For this review, take the finished solid that the model builds, in its own axes (mm). Face numbers are marked on the shaded views. A direction names the side the tool comes from. Coordinates: 2 decimals unless noted, no trailing zeros. Order: outer loops, then holes, each group sorted by start corner. A loop starts at its lowest first (then second) coordinate and runs counter-clockwise, first axis right, second up. Notation, with made-up numbers: M -18.5,33.5 L 12.5,33.5 A16 ccw 12.5,58.5 Z; hole C 30.5,-14 d5. An arc over 180 degrees is marked long. Use CSV: the item, a comma, the result in double quotes.
```python
from build123d import *

# Parameters (mm, degrees)
F0_R     = 15.875
F0_R_2   = 6.35
F1_DEPTH = 31.75
F2_DEPTH = 76.2
F3_R     = 4.445
F4_DEPTH = 76.2


with BuildPart() as f1:
    # F0 (on Top) → F1 (new body)
    with BuildSketch(Plane.XY):
        Circle(F0_R)
        Circle(F0_R_2, mode=Mode.SUBTRACT)
    extrude(amount=-F1_DEPTH)

    # F0 (on Top) → F2 (join)
    with BuildSketch(Plane.XY):
        Circle(F0_R_2)
    extrude(amount=-F2_DEPTH)

    # F3 (on Right) → F4 (join, symmetric)
    with BuildSketch(Plane.YZ):
        with Locations((0, -15.875)):
            Circle(F3_R)
    extrude(amount=F4_DEPTH, both=True)

    # F7 (on Front) → F8 (revolve)
    with BuildSketch(Plane.XZ):
        with BuildLine():
            Line((73.423605, -5.542184), (73.423605, -25.862184))
            ThreePointArc((73.423605, -25.862184), (83.583605, -15.702184), (73.423605, -5.542184))
        make_face()
    revolve(axis=Axis((73.423605, 0, -26.137914), (0, 0, -1)))



with BuildPart() as f6:
    # F5 (on Front) → F6 (revolve)
    with BuildSketch(Plane.XZ):
        with BuildLine():
            Line((-76.2, -26.452393), (-76.2, -6.132393))
            ThreePointArc((-76.2, -6.132393), (-86.36, -16.292393), (-76.2, -26.452393))
        make_face()
    revolve(axis=Axis((-76.2, 0, -32.181646), (0, 0, -1)))


with BuildPart() as f1_1:
    add(f1.part)

    add(f6.part)  # F9 merges F6
    # F5 (on Front) → F9 (revolve)
    with BuildSketch(Plane.XZ):
        with BuildLine():
            Line((-76.2, -26.452393), (-76.2, -6.132393))
            ThreePointArc((-76.2, -6.132393), (-86.36, -16.292393), (-76.2, -26.452393))
        make_face()
    revolve(axis=Axis((-76.2, 0, -32.181646), (0, 0, -1)))


solid = f1_1.part
```
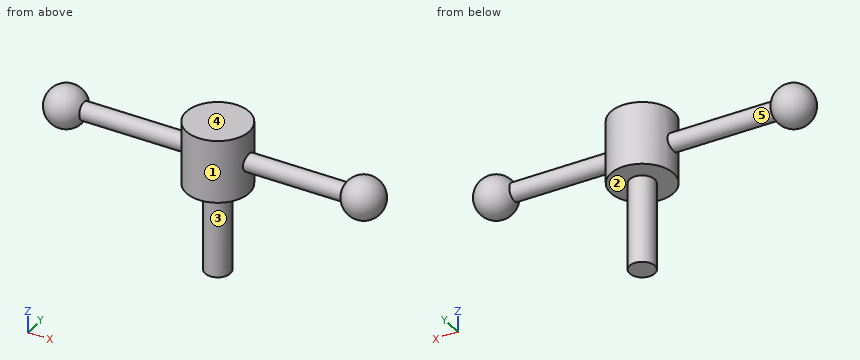
Item 1: Clearance check with flat-ended pins moving along their axes: pin 1 Ø12 at (x, z) = (65, -12) entering from -Y; pin 2 Ø6 at (x, y) = (-16.5, 1.5) entering from -Z. State where each tip first meets the part, or that it passes through.
Solutions:
pin 1,"y = -9.64"
pin 2,"z = -31.75"
Item 2: Add section B-B on y = 2. State the section outline as (x, z) points.
Solutions:
outline,"M -67.26,-11.91 A9.96 ccw long -66.89,-19.84 L -15.75,-19.84 L -15.75,-31.75 L -6.03,-31.75 L -6.03,-76.2 L 6.03,-76.2 L 6.03,-31.75 L 15.75,-31.75 L 15.75,-19.84 L 64.36,-19.84 A9.96 ccw long 64.21,-11.91 L 15.75,-11.91 L 15.75,0 L -15.75,0 L -15.75,-11.91 Z"
Item 3: To check wall thickness, follow line 1 along X through (y, z) = (7, -21); line 2 along X through (y, z) = (-0.5, -46.5); line 3 along Z through (x, y) = (5, -11). State the ranges of each line that lie inside material, in increasing order. Write a range as [from, to].
Solutions:
line 1,"[-81.86, -70.54], [-14.25, 14.25], [68.31, 78.54]"
line 2,"[-6.33, 6.33]"
line 3,"[-31.75, 0]"
Item 4: Add section C-C on z = -56. State the section outline as (x, y) points.
Solutions:
outline,"C 0,0 d12.7"
Item 5: Add section D-D on z = -23.5. State the section outline as (x, y) points (3 decimals).
Solutions:
outline,"C -76.2,0 d14.321; C 0,0 d31.75; C 73.424,0 d13.026"
Item 6: Add section A-A on x = 0. State the section outline as (y, z) points (3 decimals).
Solutions:
outline,"M -15.875,-31.75 L -6.35,-31.75 L -6.35,-76.2 L 6.35,-76.2 L 6.35,-31.75 L 15.875,-31.75 L 15.875,0 L -15.875,0 Z"
Item 7: For the marked faces 4 and 5, list the 3-axis set-ups (+Z, -Z, +X, -X, +Y, -Y) from which the entire face can be reached by the end or side of a thin tool; tool diameter is ignored.
Solutions:
face 4,"+Z, +X, -X, +Y, -Y"
face 5,"none"
Item 8: Draft analysis for pull direction X (two halves, no side actions). For the marked faces 1, 2 and 3, state which applies: released by +X, released by -X, zero draft, split by the parting line, or undercut.
Solutions:
face 1,"undercut"
face 2,"zero draft"
face 3,"split by the parting line"
